Can you work these out from the model? Positions are in its coordinate system, mm. A direction names the side the tool comes from. Round coordinates to 2 decimals unless told otherwise and drop trailing zeros. Loops run counter-clockwise (first coordinate to the right, second up) from the corner with the lowest first, then second, coordinate; pieces in that order, holes last. Notation, with made-up numbers: (76.5, -8) -> (92.5, -8) arc R17 ccw to (92.5, 3) -> close; hole circle Ø1 at (-32, 60.25). An arc over 180 degrees is marked (long way). Answer as a JSON object with one key per item and string values.
```python
from build123d import *

# Parameters (mm, degrees)
SKETCH_W      = 80.5
SKETCH_H      = 70
PAD_DEPTH     = 3
FILLET_R      = 4.5
SKETCH001_R   = 1.75
POCKET_DEPTH  = 3.001
SKETCH002_R   = 4.5
SKETCH002_R_2 = 3
PAD001_DEPTH  = 5
FILLET001_R   = 1


with BuildPart() as part:
    # Sketch → Pad (new body)
    with BuildSketch(Plane.XY):
        Rectangle(SKETCH_W, SKETCH_H)
    extrude(amount=PAD_DEPTH)

    # Fillet
    fillet_edges = [part.edges().sort_by_distance(p)[0] for p in [
        (-40.25, -35, 1.5),
        (40.25, -35, 1.5),
        (40.25, 35, 1.5),
        (-40.25, 35, 1.5),
    ]]
    fillet(fillet_edges, radius=FILLET_R)

    # Sketch001 (on Face5 of Fillet) → Pocket (cut, through all)
    with BuildSketch(Plane.XY.offset(3)):
        with Locations((-35.75, -30.5)):
            Circle(SKETCH001_R)
        with Locations((35.75, -30.5)):
            Circle(SKETCH001_R)
        with Locations((35.75, 30.5)):
            Circle(SKETCH001_R)
        with Locations((-35.75, 30.5)):
            Circle(SKETCH001_R)
    extrude(amount=-POCKET_DEPTH, mode=Mode.SUBTRACT)

    # Sketch002 (on Face5 of Pocket) → Pad001 (join)
    with BuildSketch(Plane.XY.offset(3)):
        with Locations((-35.75, 30.5)):
            Circle(SKETCH002_R)
        with Locations((-35.75, 30.5)):
            Circle(SKETCH002_R_2, mode=Mode.SUBTRACT)
        with Locations((-35.75, -30.5)):
            Circle(SKETCH002_R)
        with Locations((-35.75, -30.5)):
            Circle(SKETCH002_R_2, mode=Mode.SUBTRACT)
    pad001 = extrude(amount=PAD001_DEPTH)

    # Mirrored: Pad001 across YZ
    add(pad001.mirror(Plane.YZ))

    # Fillet001
    fillet001_edges = [part.edges().sort_by_distance(p)[0] for p in [
        (-40.25, -30.5, 8),
        (-40.25, 30.5, 8),
        (40.25, 30.5, 8),
        (40.25, -30.5, 8),
    ]]
    fillet(fillet001_edges, radius=FILLET001_R)


solid = part.part
```
Q1. We'd pull the mould along Y, two halves only. Please class faces 1 (the flat face through (-1, -35, 1)), 2 (the cylindrical face through (-34.133, 29.83, 1.521)), 3 (the cylindrical face through (-34.133, -31.17, 1.521)), 4 (the flat face through (-1, 0, 0)): pulls with the +Y half, pulls with the -Y half, needs draft (parallel to the pull), parting line crosses it, or undercut.
Determined:
{"face 1": "pulls with the -Y half", "face 2": "undercut", "face 3": "undercut", "face 4": "needs draft"}
Q2. I'm going to push flat-ended pins straight in: pin 1 (1 mm diameter, centred on x = -21.5, y = 4, fed in from +Z); pin 2 (5 mm diameter, centred on x = 35, y = -31, fed in from +Z). Where does each tip first touch, or does it pass through?
Determined:
{"pin 1": "z = 3", "pin 2": "z = 8"}
Q3. I want a section at C-C, the plane x = 17.5. Write out the boundary of the cut face in (y, z), then the cut area to 3 significant figures.
Determined:
{"outline": "(-35, 0) -> (35, 0) -> (35, 3) -> (-35, 3) -> close", "area": "210 mm²"}
Q4. If I drill on L1, parallel to Y at x = -35.75, z = 4.6; L2, parallel to Z at x = 3.5, y = -2.5; L3, parallel to Y at x = 37, z = 7.5, over which ranges is the centre line in solid material (lowest first)? Write a range as [from, to].
Determined:
{"L1": "[-35, -33.5], [-27.5, -26], [26, 27.5], [33.5, 35]", "L2": "[0, 3]", "L3": "[-34.68, -33.23], [-27.77, -26.32], [26.32, 27.77], [33.23, 34.68]"}
Q5. I want a section at A-A, the plane z = 4. Write out the boundary of the cut face in (x, y).
Determined:
{"outline": "circle Ø9 at (-35.75, -30.5); circle Ø9 at (-35.75, 30.5); circle Ø9 at (35.75, -30.5); circle Ø9 at (35.75, 30.5); hole circle Ø6 at (-35.75, -30.5); hole circle Ø6 at (-35.75, 30.5); hole circle Ø6 at (35.75, -30.5); hole circle Ø6 at (35.75, 30.5)"}
Q6. I want a section at B-B, the plane y = -7. Write out the boundary of the cut face in (x, z).
Determined:
{"outline": "(-40.25, 0) -> (40.25, 0) -> (40.25, 3) -> (-40.25, 3) -> close"}
Q7. On a 3-axis mill with a long thin cutter (end or side, diameter ignored), from which of +Z, -Z, +X, -X, +Y, -Y can I reach the whole of each face in a straight line? I mean faces 5 (the flat face through (-1, 35, 1)), 6 (the flat face through (-34, -32, 3)). Say none if no direction works.
Determined:
{"face 5": "+Z, -Z, +X, -X, +Y", "face 6": "+Z"}
